```python
from build123d import *

# Parameters (mm, degrees)
PAD003_DEPTH         = 10
SKETCH004_R          = 1
POCKET_DEPTH         = 10.001
SKETCH006_R          = 1.95
POCKET002_DEPTH      = 20.951
SKETCH007_R          = 1.95
POCKET003_DEPTH      = 100
POCKET003_DEPTH_BACK = 100


with BuildPart() as part:
    # Sketch003 → Pad003 (new body)
    with BuildSketch(Plane.XY):
        with BuildLine():
            ThreePointArc((-30.857374, -12.25), (0, -33.2), (30.857374, -12.25))
            Line((-30.857374, -12.25), (30.857374, -12.25))
        make_face()
    extrude(amount=PAD003_DEPTH)

    # Sketch004 (on Face4 of Pad003) → Pocket (cut, through all)
    with BuildSketch(Plane.XY.offset(10)):
        with Locations((4, -17.2)):
            Circle(SKETCH004_R)
        with Locations((19.8, -17.2)):
            Circle(SKETCH004_R)
        with Locations((-4, -16.9)):
            Circle(SKETCH004_R)
        with Locations((-19.8, -16.9)):
            Circle(SKETCH004_R)
    extrude(amount=-POCKET_DEPTH, mode=Mode.SUBTRACT)

    # Sketch006 (on Face2 of Pocket) → Pocket002 (cut, through all)
    with BuildSketch(Plane(origin=(0, -12.25, 0), x_dir=(-1, 0, 0), z_dir=(0, 1, 0))):
        with Locations((0, 5)):
            Circle(SKETCH006_R)
    extrude(amount=-POCKET002_DEPTH, mode=Mode.SUBTRACT)

    # Sketch007 → Pocket003 (cut, two sides)
    with BuildSketch(Plane.YZ) as pocket003_sk:
        with Locations((-20.825799, 5)):
            Circle(SKETCH007_R)
    extrude(amount=-POCKET003_DEPTH, mode=Mode.SUBTRACT)
    extrude(pocket003_sk.sketch, amount=POCKET003_DEPTH_BACK, mode=Mode.SUBTRACT)


solid = part.part
```
Build history of the part. All positions in model axes, mm. Give positions to 0.01 mm unless a question says otherwise; leave off trailing zeros. Loops run counter-clockwise (first coordinate to the right, second up) from the corner with the lowest first, then second, coordinate; pieces in that order, holes last. Notation, with made-up numbers: (61, 5.5) - (83, 5.5) arc R17 cw to (83, 31.5) - close; hole circle Ø7 at (48.5, -27). An arc over 180 degrees is marked (long way). Use a Markdown table: item, result.
(1) Band-saw the part on C-C (z = 9). Give the cut face in (x, y).
Taken from the geometry:
| item | result |
|---|---|
| outline | (-30.86, -12.25) arc R33.2 ccw to (30.86, -12.25) - close; hole circle Ø2 at (-19.8, -16.9); hole circle Ø2 at (-4, -16.9); hole circle Ø2 at (4, -17.2); hole circle Ø2 at (19.8, -17.2) |
(2) Pull direction Y, two halves, no side cores. Call faces 1 (the face through (-20.8, -16.9, 5.1)), 2 (the face through (0, -20, 10)), 3 (the face through (-0.554, -33.195, 2.708)), 4 (the face through (13.465, -18.966, 5.586)): +Y half, -Y half, draft (parallel to the pull), parting line (faces both ways), or undercut.
Taken from the geometry:
| item | result |
|---|---|
| face 1 | undercut |
| face 2 | draft |
| face 3 | -Y half |
| face 4 | undercut |
(3) Band-saw the part on D-D (x = 1). Give the cut face in (y, z), and give its area (3 significant figures).
Taken from the geometry:
| item | result |
|---|---|
| outline | (-33.18, 0) - (-12.25, 0) - (-12.25, 3.33) - (-19.83, 3.33) arc R1.95 cw to (-21.83, 3.33) - (-33.18, 3.33) - close; (-33.18, 6.67) - (-21.83, 6.67) arc R1.95 cw to (-19.83, 6.67) - (-12.25, 6.67) - (-12.25, 10) - (-33.18, 10) - close |
| area | 139 mm2 |
(4) Band-saw the part on B-B (y = -21.75). Give the cut face in (x, z).
Taken from the geometry:
| item | result |
|---|---|
| outline | (-25.08, 0) - (25.08, 0) - (25.08, 3.28) - (0.92, 3.28) arc R1.95 cw to (-0.92, 3.28) - (-25.08, 3.28) - close; (-25.08, 6.72) - (-0.92, 6.72) arc R1.95 cw to (0.92, 6.72) - (25.08, 6.72) - (25.08, 10) - (-25.08, 10) - close |
(5) Wall check: line 1 along Y through (x, z) = (-4, 4.75); line 2 along Z through (x, y) = (0, -29.75); line 3 along X through (y, z) = (-18, 3.25). Give the ranges that are in metal, low to high.
Taken from the geometry:
| item | result |
|---|---|
| line 1 | -32.96 to -22.76, -18.89 to -17.9, -15.9 to -12.25 |
| line 2 | 0 to 3.05, 6.95 to 10 |
| line 3 | -27.9 to -0.86, 0.86 to 3.4, 4.6 to 19.2, 20.4 to 27.9 |
(6) Band-saw the part on A-A (x = 19.8). Give the cut face in (y, z), and give its area (3 significant figures).
Taken from the geometry:
| item | result |
|---|---|
| outline | (-26.65, 0) - (-18.2, 0) - (-18.2, 10) - (-26.65, 10) - close; (-16.2, 0) - (-12.25, 0) - (-12.25, 10) - (-16.2, 10) - close; hole circle Ø3.9 at (-20.83, 5) |
| area | 112 mm2 |
(7) Drop flat-ended pins along their axis: pin 1 Ø1.5 at (x, z) = (2.5, 2.5) entering from -Y; pin 2 Ø5 at (y, z) = (-20.83, 5) entering from -X; pin 3 Ø4 at (y, z) = (-22.5, 4.5) entering from -X. Give the stop position or say it passes through.
Taken from the geometry:
| item | result |
|---|---|
| pin 1 | y = -33.15 |
| pin 2 | x = -27.68 |
| pin 3 | x = -25.63 |
